from build123d import *

# Parameters (mm, degrees)
SKETCH1_R          = 3.175
SKETCH1_R_2        = 1.778
BASE_FLANGE1_DEPTH = 5.588
FILLET1_R          = 6.35
CUT_EXTRUDE2_REACH = 196.352
SKETCH3_R          = 3.96875


# Sheet-metal steps are written as plain solids
with BuildPart() as part:
    # Sketch1 → Base-Flange1 (new body)
    with BuildSketch(Plane(origin=(0, 0, 0), x_dir=(1, 0, 0), z_dir=(0, 1, 0))):
        Polygon((-102.488290128, 43.05937504), (-102.488290128, -165.037938429), (-26.750144364, -165.037938429), (-26.750144364, -96.438243977), (35.245709983, -96.438243977), (35.245709983, -43.059375352), (102.488290128, -43.059375352), (102.488290128, 120.582488744), (26.754290128, 120.582488744), (26.754290128, 96.438243353), (-35.245709872, 96.438243353), (-35.245709872, 43.05937504), align=None)
        with Locations(Location((-37.754290017, -153.305196741, 0), (0, 0, 270))):
            Circle(SKETCH1_R, mode=Mode.SUBTRACT)
        with Locations(Location((-37.754290017, -52.76904616, 0), (0, 0, 270))):
            Circle(SKETCH1_R, mode=Mode.SUBTRACT)
        with Locations(Location((37.754290128, 10.201797316, 0), (0, 0, 270))):
            Circle(SKETCH1_R, mode=Mode.SUBTRACT)
        with Locations(Location((37.754290128, 110.737947896, 0), (0, 0, 270))):
            Circle(SKETCH1_R, mode=Mode.SUBTRACT)
        with Locations(Location((95.814087341, 93.888699503, 0), (0, 0, 270))):
            Circle(SKETCH1_R_2, mode=Mode.SUBTRACT)
        with Locations(Location((75.428905946, 95.223880898, 0), (0, 0, 270))):
            Circle(SKETCH1_R_2, mode=Mode.SUBTRACT)
        with Locations(Location((75.428905946, 68.283112535, 0), (0, 0, 270))):
            Circle(SKETCH1_R_2, mode=Mode.SUBTRACT)
        with Locations(Location((95.814087341, 69.61829393, 0), (0, 0, 270))):
            Circle(SKETCH1_R_2, mode=Mode.SUBTRACT)
        with Locations(Location((95.814087341, 12.135202787, 0), (0, 0, 270))):
            Circle(SKETCH1_R_2, mode=Mode.SUBTRACT)
        with Locations(Location((95.814087341, -12.135202787, 0), (0, 0, 270))):
            Circle(SKETCH1_R_2, mode=Mode.SUBTRACT)
        with Locations(Location((75.428905946, 13.470384182, 0), (0, 0, 270))):
            Circle(SKETCH1_R_2, mode=Mode.SUBTRACT)
        with Locations(Location((75.428905946, -13.470384182, 0), (0, 0, 270))):
            Circle(SKETCH1_R_2, mode=Mode.SUBTRACT)
        with Locations(Location((-95.814087341, 12.135202787, 0), (0, 0, 270))):
            Circle(SKETCH1_R_2, mode=Mode.SUBTRACT)
        with Locations(Location((-75.428905946, 13.470384182, 0), (0, 0, 270))):
            Circle(SKETCH1_R_2, mode=Mode.SUBTRACT)
        with Locations(Location((-75.428905946, -13.470384182, 0), (0, 0, 270))):
            Circle(SKETCH1_R_2, mode=Mode.SUBTRACT)
        with Locations(Location((-95.814087341, -12.135202787, 0), (0, 0, 270))):
            Circle(SKETCH1_R_2, mode=Mode.SUBTRACT)
        with Locations(Location((-95.814087341, -69.61829393, 0), (0, 0, 270))):
            Circle(SKETCH1_R_2, mode=Mode.SUBTRACT)
        with Locations(Location((-75.428905946, -68.283112535, 0), (0, 0, 270))):
            Circle(SKETCH1_R_2, mode=Mode.SUBTRACT)
        with Locations(Location((-75.428905946, -95.223880898, 0), (0, 0, 270))):
            Circle(SKETCH1_R_2, mode=Mode.SUBTRACT)
        with Locations(Location((-95.814087341, -93.888699503, 0), (0, 0, 270))):
            Circle(SKETCH1_R_2, mode=Mode.SUBTRACT)
    extrude(amount=-BASE_FLANGE1_DEPTH)

    # Fillet1
    fillet1_edges = [part.edges().sort_by_distance(p)[0] for p in [
        (-35.245709872, -2.794, -43.05937504),
        (-35.245709872, -2.794, -96.438243353),
        (26.754290128, -2.794, -96.438243353),
        (26.754290128, -2.794, -120.582488744),
        (102.488290128, -2.794, -120.582488744),
        (102.488290128, -2.794, 43.059375352),
        (35.245709983, -2.794, 43.059375352),
        (35.245709983, -2.794, 96.438243977),
        (-26.750144364, -2.794, 96.438243977),
        (-26.750144364, -2.794, 165.037938429),
        (-102.488290128, -2.794, 165.037938429),
        (-102.488290128, -2.794, -43.05937504),
    ]]
    fillet(fillet1_edges, radius=FILLET1_R)

    # Sketch3 → Cut-Extrude2 (cut, up to next)
    with BuildSketch(Plane(origin=(0, 0, 0), x_dir=(1, 0, 0), z_dir=(0, 1, 0)), mode=Mode.PRIVATE) as cut_extrude2_sk1:
        with Locations(Location((-93.33196009, 33.903045002, 0), (0, 0, 270))):
            Circle(SKETCH3_R)
    cut_extrude2_tool1 = extrude(cut_extrude2_sk1.sketch, amount=-CUT_EXTRUDE2_REACH, mode=Mode.PRIVATE) & part.part
    # Sketch3 → Cut-Extrude2 (cut, up to next)
    with BuildSketch(Plane(origin=(0, 0, 0), x_dir=(1, 0, 0), z_dir=(0, 1, 0)), mode=Mode.PRIVATE) as cut_extrude2_sk2:
        with Locations(Location((-93.33196009, -155.881608392, 0), (0, 0, 270))):
            Circle(SKETCH3_R)
    cut_extrude2_tool2 = extrude(cut_extrude2_sk2.sketch, amount=-CUT_EXTRUDE2_REACH, mode=Mode.PRIVATE) & part.part
    # Sketch3 → Cut-Extrude2 (cut, up to next)
    with BuildSketch(Plane(origin=(0, 0, 0), x_dir=(1, 0, 0), z_dir=(0, 1, 0)), mode=Mode.PRIVATE) as cut_extrude2_sk3:
        with Locations(Location((93.33196009, 111.426158707, 0), (0, 0, 270))):
            Circle(SKETCH3_R)
    cut_extrude2_tool3 = extrude(cut_extrude2_sk3.sketch, amount=-CUT_EXTRUDE2_REACH, mode=Mode.PRIVATE) & part.part
    # Sketch3 → Cut-Extrude2 (cut, up to next)
    with BuildSketch(Plane(origin=(0, 0, 0), x_dir=(1, 0, 0), z_dir=(0, 1, 0)), mode=Mode.PRIVATE) as cut_extrude2_sk4:
        with Locations(Location((93.33196009, -33.903045314, 0), (0, 0, 270))):
            Circle(SKETCH3_R)
    cut_extrude2_tool4 = extrude(cut_extrude2_sk4.sketch, amount=-CUT_EXTRUDE2_REACH, mode=Mode.PRIVATE) & part.part
    add(cut_extrude2_tool1.solids().sort_by_distance((-93.33196, 0, -33.903045))[0], mode=Mode.SUBTRACT)
    add(cut_extrude2_tool2.solids().sort_by_distance((-93.33196, 0, 155.881608))[0], mode=Mode.SUBTRACT)
    add(cut_extrude2_tool3.solids().sort_by_distance((93.33196, 0, -111.426159))[0], mode=Mode.SUBTRACT)
    add(cut_extrude2_tool4.solids().sort_by_distance((93.33196, 0, 33.903045))[0], mode=Mode.SUBTRACT)


solid = part.part
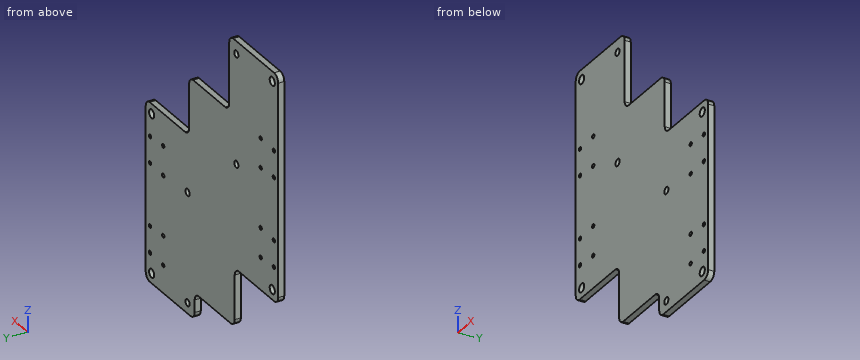
Design review of the part built by this model. Coordinates are the model's own, in mm. Give positions to 0.01 mm unless a question says otherwise; leave off trailing zeros. Order: outer loops, then holes, each group sorted by start corner. A loop starts at its lowest first (then second) coordinate and runs counter-clockwise, first axis right, second up. Notation, with made-up numbers: (10.25, 86.5) - (21.25, 86.5) arc R3 cw to (21.25, 91.5) - close; hole circle Ø5 at (77, -35.75). An arc over 180 degrees is marked (long way). Write item = value, one per line. Start each with the question number.
Q1. Clearance check with flat-ended pins moving along their axes: pin 1 Ø3 at (x, y) = (71, -2) entering from +Z; pin 2 Ø3 at (y, z) = (-1.5, 64) entering from +X; pin 3 Ø3 at (x, y) = (-34.5, -1.5) entering from -Z. State where each tip first meets the part, or that it passes through.
Q2. To check wall thickness, follow L1, parallel to X at y = -1.3, z = 153.5; L2, parallel to X at y = -3.6, z = 85; L3, parallel to Z at x = 2, y = -3.1. State the ranges of each line that lie inside material, in increasing order. Write a range as from..to.
Q3. We need section C-C on y = -2.15. State how many separate pieces and enclosed holes the cut face has, plus the area to 3 significant figures.
Q4. We need section B-B on x = 17.5. State the section outline as (y, z) points.
Q5. We need section A-A on z = -78. State the section outline as (x, y) points, plus the area to 3 significant figures.
Working result:
q1.pin_1 = 43.06
q1.pin_2 = 35.25
q1.pin_3 = -94.93
q2.L1 = -102.49..-96.51, -90.16..-40.92, -34.59..-26.75
q2.L2 = -102.49..35.25
q2.L3 = -96.44..96.44
q3.separate_pieces = 1
q3.enclosed_holes = 24
q3.area = 38,900 mm²
q4.outline = (-5.59, -96.44) - (0, -96.44) - (0, 96.44) - (-5.59, 96.44) - close
q5.outline = (-35.25, -5.59) - (102.49, -5.59) - (102.49, 0) - (-35.25, 0) - close
q5.area = 770 mm²
